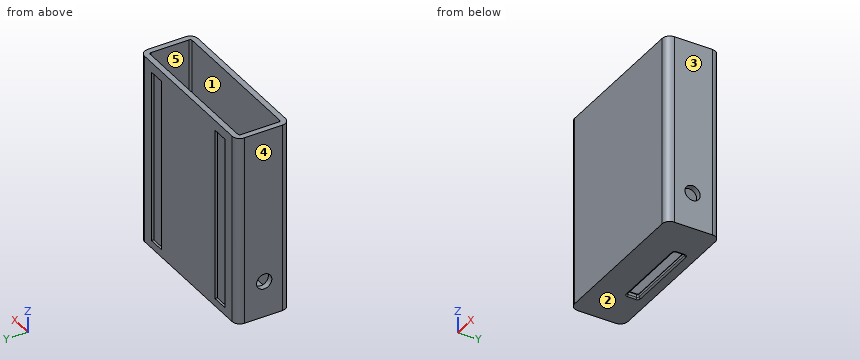
Autodesk Fusion 360 part; units mm, degrees
sketch "Sketch1" plane through (0, 0, 0) normal (0, 0, 1) x (1, 0, 0)
  line L0 (22.7481, 79.1534) -> (232.7481, 79.1534)
  line L1 (232.7481, 79.1534) -> (232.7481, 9.1534)
  line L2 (232.7481, 9.1534) -> (22.7481, 9.1534)
  line L3 (22.7481, 9.1534) -> (22.7481, 79.1534)
extrude "Extrude1" add sketch "Sketch1" along normal blind 250
fillet "Fillet1" radius 10 1 edges at (22.7481, 9.1534, 125)
fillet "Fillet2" radius 10 1 edges at (232.7481, 9.1534, 125)
fillet "Fillet3" radius 10 1 edges at (22.7481, 79.1534, 125)
fillet "Fillet4" radius 10 1 edges at (232.7481, 79.1534, 125)
shell "Shell1" thickness 7.5 removed faces 1 at (159.4147, 32.4867, 250)
sketch "Sketch2" plane through (0, 0, 0) normal (0, 0, 1) x (1, 0, 0)
  line L0 (180.4304, 50.4408) -> (77.6973, 50.4408)
  line L1 (77.6973, 50.4408) -> (77.6973, 65.4408)
  line L2 (77.6973, 65.4408) -> (180.4304, 65.4408)
  line L3 (180.4304, 65.4408) -> (180.4304, 50.4408)
  line L4 (180.4304, 50.4408) -> (77.6973, 65.4408) construction
  line L5 (77.6973, 50.4408) -> (180.4304, 65.4408) construction
  point P0 (129.0638, 57.9408)
extrude "Extrude2" cut sketch "Sketch2" along normal blind 24
fillet "Fillet5" radius 2 12 edges at (129.0638, 65.4408, 0) (129.0638, 50.4408, 0) (77.6973, 57.9408, 0) (180.4304, 57.9408, 0) (77.6973, 50.4408, 3.75) (129.0638, 65.4408, 7.5) (77.6973, 57.9408, 7.5) (77.6973, 65.4408, 3.75) (180.4304, 50.4408, 3.75) (180.4304, 65.4408, 3.75) (180.4304, 57.9408, 7.5) (129.0638, 50.4408, 7.5) 4 faces at (77.6973, 55.4408, 2.5) (146.186, 50.4408, 2.5) (180.4304, 60.4408, 5) (111.9416, 65.4408, 2.5)
sketch "Sketch3" plane through (0, 0, 0) normal (0, 0, -1) x (1, 0, 0)
  arc A0 (222.7481, -79.1534) -> (232.7481, -69.1534) centre (222.7481, -69.1534) ccw
  line L0 (232.7481, -69.1534) -> (232.7481, -19.1534)
  arc A1 (232.7481, -19.1534) -> (222.7481, -9.1534) centre (222.7481, -19.1534) ccw
  line L1 (222.7481, -9.1534) -> (32.7481, -9.1534)
  arc A2 (32.7481, -9.1534) -> (22.7481, -19.1534) centre (32.7481, -19.1534) ccw
  line L2 (22.7481, -19.1534) -> (22.7481, -69.1534)
  arc A3 (22.7481, -69.1534) -> (32.7481, -79.1534) centre (32.7481, -69.1534) ccw
  line L3 (32.7481, -79.1534) -> (222.7481, -79.1534)
  arc A4 (178.4304, -67.4408) -> (182.4304, -63.4408) centre (178.4304, -63.4408) ccw
  line L4 (178.4304, -67.4408) -> (79.6973, -67.4408)
  arc A5 (75.6973, -63.4408) -> (79.6973, -67.4408) centre (79.6973, -63.4408) ccw
  line L5 (75.6973, -63.4408) -> (75.6973, -52.4408)
  arc A6 (79.6973, -48.4408) -> (75.6973, -52.4408) centre (79.6973, -52.4408) ccw
  line L6 (79.6973, -48.4408) -> (178.4304, -48.4408)
  arc A7 (182.4304, -52.4408) -> (178.4304, -48.4408) centre (178.4304, -52.4408) ccw
  line L7 (182.4304, -52.4408) -> (182.4304, -63.4408)
hole "Hole1" at (22.7481, 43.0604, 47.3957) direction (1, 0, 0) diameter 20 depth 300 tip angle 118
ref_plane "WorkPlane1" through (127.7481, 79.1534, 125) normal (0, 1, 0) x (-1, 0, 0)
sketch "Sketch4" plane through (0, 79.1534, 0) normal (0, 1, 0) x (1, 0, 0)
  line L0 (207.7481, -10) -> (185.6481, -10)
  line L1 (185.6481, -10) -> (185.6481, -237)
  line L2 (185.6481, -237) -> (207.7481, -237)
  line L3 (207.7481, -237) -> (207.7481, -10)
  line L4 (32.7481, 0) -> (222.7481, 0)
  line L5 (222.7481, 0) -> (222.7481, -250)
  line L6 (207.7481, -10) -> (185.6481, -10)
  line L7 (185.6481, -10) -> (185.6481, -237)
  line L8 (185.6481, -237) -> (207.7481, -237)
  line L9 (207.7481, -237) -> (207.7481, -10)
  line L10 (69.8481, -10) -> (47.7481, -10)
  line L11 (47.7481, -10) -> (47.7481, -237)
  line L12 (47.7481, -237) -> (69.8481, -237)
  line L13 (69.8481, -237) -> (69.8481, -10)
  line L14 (32.7481, -250) -> (32.7481, 0)
  dimension "d25" = 10
  dimension "d26" = 15
  dimension "d27" = 22.1
  dimension "d28" = 227
  dimension "d29" = 227
  dimension "d30" = 22.1
  dimension "d31" = 10
  dimension "d32" = 15
extrude "Extrude3" cut sketch "Sketch4" against normal blind 3
Model file for the job. Use its own axes, mm. Face numbers are marked on the shaded views. A direction names the side the tool comes from. Give positions to 0.01 mm unless a question says otherwise; leave off trailing zeros. Write each loop counter-clockwise with the first axis right and the second up, starting at its lowest first coordinate (ties: lowest second). Pieces come first, ordered by that corner, then holes. Notation, with made-up numbers: M -12.75,10 L 31.25,10 A29 ccw 31.25,42 Z; hole C -21,46 d2. An arc over 180 degrees is marked long. Use a Markdown table: item, result.
1) Pin check, flat tips, straight feed: pin 1 (1.5 mm diameter, centred on y = 78, z = 87, fed in from -X); pin 2 (12 mm diameter, centred on x = 110.5, y = 46.5, fed in from +Z); pin 3 (2.5 mm diameter, centred on y = 77.5, z = 160, fed in from +X); pin 4 (18 mm diameter, centred on y = 43.06, z = 47.4, fed in from +X). Stop position of each tip, or through.
Responses:
| item | result |
|---|---|
| pin 1 | stops at x = 26.88 |
| pin 2 | stops at z = 7.5 |
| pin 3 | stops at x = 229.79 |
| pin 4 | passes through |
2) Cut at B-B (y = 58). List the corners of the cut face in (x, z), and give its area (3 significant figures).
Responses:
| item | result |
|---|---|
| outline | M 22.75,0 L 75.7,0 A2 ccw 77.7,2 L 77.7,5.5 A2 ccw 75.7,7.5 L 30.25,7.5 L 30.25,250 L 22.75,250 Z; M 180.43,2 A2 ccw 182.43,0 L 232.75,0 L 232.75,250 L 225.25,250 L 225.25,7.5 L 182.43,7.5 A2 ccw 180.43,5.5 Z |
| area | 4,440 mm2 |
3) Drill centre lines: line 1 (Y direction, x = 110.5, z = 120); line 2 (X direction, y = 32, z = 42.5); line 3 (Y direction, x = 62, z = 170). Where is each one in solid material? Low to high. Write a range as from..to.
Responses:
| item | result |
|---|---|
| line 1 | y = 9.15..16.65, 71.65..79.15 |
| line 2 | x = 22.75..30.25, 225.25..232.75 |
| line 3 | y = 9.15..16.65, 71.65..76.15 |
4) Cut at D-D (x = 51.5). List the corners of the cut face in (y, z), and give its area (3 significant figures).
Responses:
| item | result |
|---|---|
| outline | M 9.15,0 L 79.15,0 L 79.15,10 L 76.15,10 L 76.15,237 L 79.15,237 L 79.15,250 L 71.65,250 L 71.65,7.5 L 16.65,7.5 L 16.65,250 L 9.15,250 Z |
| area | 3,480 mm2 |
5) Cut at A-A (x = 119). List the corners of the cut face in (y, z), and give its area (3 significant figures).
Responses:
| item | result |
|---|---|
| outline | M 9.15,0 L 48.44,0 A2 ccw 50.44,2 L 50.44,5.5 A2 ccw 48.44,7.5 L 16.65,7.5 L 16.65,250 L 9.15,250 Z; M 65.44,2 A2 ccw 67.44,0 L 79.15,0 L 79.15,250 L 71.65,250 L 71.65,7.5 L 67.44,7.5 A2 ccw 65.44,5.5 Z |
| area | 4,050 mm2 |
6) Pull direction X, two halves, no side cores. Call the marked faces 1, 2 and 3: +X half, -X half, draft (parallel to the pull), parting line (faces both ways), or undercut.
Responses:
| item | result |
|---|---|
| face 1 | undercut |
| face 2 | draft |
| face 3 | +X half |
7) Tool access for the marked faces 4 and 5: list every direction of +Z, -Z, +X, -X, +Y, -Y with a clear straight run to the whole face (end or side of a thin tool).
Responses:
| item | result |
|---|---|
| face 4 | +Z, -Z, -X, +Y, -Y |
| face 5 | +Z |
8) Cut at C-C (z = 76). List the corners of the cut face in (x, y).
Responses:
| item | result |
|---|---|
| outline | M 22.75,19.15 A10 ccw 32.75,9.15 L 222.75,9.15 A10 ccw 232.75,19.15 L 232.75,69.15 A10 ccw 222.75,79.15 L 207.75,79.15 L 207.75,76.15 L 185.65,76.15 L 185.65,79.15 L 69.85,79.15 L 69.85,76.15 L 47.75,76.15 L 47.75,79.15 L 32.75,79.15 A10 ccw 22.75,69.15 Z; hole M 30.25,19.15 A2.5 ccw 32.75,16.65 L 222.75,16.65 A2.5 ccw 225.25,19.15 L 225.25,69.15 A2.5 ccw 222.75,71.65 L 32.75,71.65 A2.5 ccw 30.25,69.15 Z |
